Can you work these out from the model? Positions are in its coordinate system, mm. A direction names the side the tool comes from. Round coordinates to 2 decimals unless told otherwise and drop trailing zeros. Order: outer loops, then holes, each group sorted by start corner. A loop starts at its lowest first (then second) coordinate and runs counter-clockwise, first axis right, second up. Notation, with made-up numbers: (-4.75, -30) -> (2.25, -30) arc R14 ccw to (2.25, -10) -> close; hole circle Ø10 at (35.25, -13). An arc over 180 degrees is marked (long way). Use a Markdown table: item, result. Add a question column.
Q1. We'd pull the mould along X, two halves only. Please class faces 3 (the face through (0, -10, 2)), 4 (the face through (-42.15, 11.99, 2.41)), 5 (the face through (4, 15, 2)): +X half, -X half, draft (parallel to the pull), parting line (faces both ways), or undercut.
Q2. For faces 1 (the face through (45, 0, 2)), 2 (the face through (-19.25, 0, 2)), which set-ups out of +Z, -Z, +X, -X, +Y, -Y let a thin tool reach every point of the face, with its end or its side?
Q3. If we section it at B-B on z = 1.5: Give the number of separate pieces and of enclosed holes in the cut face, plus the area to 3 significant figures.
Q4. I need wall thicknesses on line 1 along Y through (x, z) = (37.5, 1.5); line 2 along Y through (x, z) = (24.56, 3.4); line 3 along X through (y, z) = (9.5, 3.2). Which ranges of each line are inside material? Lowest first, please. Write a range as [from, to].
Q5. If we section it at A-A on x = 16: List the corners of the cut face in (y, z) for me, plus the area to 3 significant figures.
```python
from build123d import *

# Parameters (mm, degrees)
ESQUISSE1_W             = 90
ESQUISSE1_H             = 30
BOSS_EXTRU_1_DEPTH      = 4.7625
CONG_1_R                = 10
ESQUISSE2_R             = 6.35
ENL_V_MAT_EXTRU_1_DEPTH = 6
ENL_V_MAT_EXTRU_2_REACH = 49.673
ESQUISSE3_W             = 40
ESQUISSE3_H             = 20
CONG_2_R                = 1.27
ENL_V_MAT_EXTRU_3_REACH = 49.673
ESQUISSE4_R             = 1.09
ENL_V_MAT_EXTRU_4_REACH = 49.673
ESQUISSE6_R             = 1.5


with BuildPart() as part:
    # Esquisse1 → Boss.-Extru.1 (new body)
    with BuildSketch(Plane.XY):
        Rectangle(ESQUISSE1_W, ESQUISSE1_H)
    extrude(amount=BOSS_EXTRU_1_DEPTH)

    # Congé1
    cong_1_edges = [part.edges().sort_by_distance(p)[0] for p in [
        (-45, -15, 2.38125),
        (-45, 15, 2.38125),
    ]]
    fillet(cong_1_edges, radius=CONG_1_R)

    # Esquisse2 → Enlèv. mat.-Extru.1 (cut)
    with BuildSketch(Plane.XY.offset(4.7625)):
        with Locations((-35, 0)):
            Circle(ESQUISSE2_R)
    extrude(amount=-ENL_V_MAT_EXTRU_1_DEPTH, mode=Mode.SUBTRACT)

    # Esquisse3 → Enlèv. mat.-Extru.2 (cut, up to next)
    with BuildSketch(Plane.XY.offset(4.7625), mode=Mode.PRIVATE) as enl_v_mat_extru_2_sk1:
        with Locations((0.75, 0)):
            Rectangle(ESQUISSE3_W, ESQUISSE3_H)
    enl_v_mat_extru_2_tool1 = extrude(enl_v_mat_extru_2_sk1.sketch, amount=-ENL_V_MAT_EXTRU_2_REACH, mode=Mode.PRIVATE) & part.part
    add(enl_v_mat_extru_2_tool1.solids().sort_by_distance((0.75, 0, 4.7625))[0], mode=Mode.SUBTRACT)

    # Congé2
    cong_2_edges = [part.edges().sort_by_distance(p)[0] for p in [
        (-19.25, -10, 2.38125),
        (-19.25, 10, 2.38125),
        (20.75, 10, 2.38125),
        (20.75, -10, 2.38125),
    ]]
    fillet(cong_2_edges, radius=CONG_2_R)

    # Esquisse4 → Enlèv. mat.-Extru.3 (cut, up to next)
    with BuildSketch(Plane.XY.offset(4.7625), mode=Mode.PRIVATE) as enl_v_mat_extru_3_sk1:
        with Locations((-23.06, 5.19)):
            Circle(ESQUISSE4_R)
    enl_v_mat_extru_3_tool1 = extrude(enl_v_mat_extru_3_sk1.sketch, amount=-ENL_V_MAT_EXTRU_3_REACH, mode=Mode.PRIVATE) & part.part
    # Esquisse4 → Enlèv. mat.-Extru.3 (cut, up to next)
    with BuildSketch(Plane.XY.offset(4.7625), mode=Mode.PRIVATE) as enl_v_mat_extru_3_sk2:
        with Locations((-23.06, -5.19)):
            Circle(ESQUISSE4_R)
    enl_v_mat_extru_3_tool2 = extrude(enl_v_mat_extru_3_sk2.sketch, amount=-ENL_V_MAT_EXTRU_3_REACH, mode=Mode.PRIVATE) & part.part
    # Esquisse4 → Enlèv. mat.-Extru.3 (cut, up to next)
    with BuildSketch(Plane.XY.offset(4.7625), mode=Mode.PRIVATE) as enl_v_mat_extru_3_sk3:
        with Locations((24.56, -5.19)):
            Circle(ESQUISSE4_R)
    enl_v_mat_extru_3_tool3 = extrude(enl_v_mat_extru_3_sk3.sketch, amount=-ENL_V_MAT_EXTRU_3_REACH, mode=Mode.PRIVATE) & part.part
    # Esquisse4 → Enlèv. mat.-Extru.3 (cut, up to next)
    with BuildSketch(Plane.XY.offset(4.7625), mode=Mode.PRIVATE) as enl_v_mat_extru_3_sk4:
        with Locations((24.56, 5.19)):
            Circle(ESQUISSE4_R)
    enl_v_mat_extru_3_tool4 = extrude(enl_v_mat_extru_3_sk4.sketch, amount=-ENL_V_MAT_EXTRU_3_REACH, mode=Mode.PRIVATE) & part.part
    add(enl_v_mat_extru_3_tool1.solids().sort_by_distance((-23.06, 5.19, 4.7625))[0], mode=Mode.SUBTRACT)
    add(enl_v_mat_extru_3_tool2.solids().sort_by_distance((-23.06, -5.19, 4.7625))[0], mode=Mode.SUBTRACT)
    add(enl_v_mat_extru_3_tool3.solids().sort_by_distance((24.56, -5.19, 4.7625))[0], mode=Mode.SUBTRACT)
    add(enl_v_mat_extru_3_tool4.solids().sort_by_distance((24.56, 5.19, 4.7625))[0], mode=Mode.SUBTRACT)

    # Esquisse6 → Enlèv. mat.-Extru.4 (cut, up to next)
    with BuildSketch(Plane.XY.offset(4.7625), mode=Mode.PRIVATE) as enl_v_mat_extru_4_sk1:
        with Locations((37.5, 10)):
            Circle(ESQUISSE6_R)
    enl_v_mat_extru_4_tool1 = extrude(enl_v_mat_extru_4_sk1.sketch, amount=-ENL_V_MAT_EXTRU_4_REACH, mode=Mode.PRIVATE) & part.part
    # Esquisse6 → Enlèv. mat.-Extru.4 (cut, up to next)
    with BuildSketch(Plane.XY.offset(4.7625), mode=Mode.PRIVATE) as enl_v_mat_extru_4_sk2:
        with Locations((37.5, -10)):
            Circle(ESQUISSE6_R)
    enl_v_mat_extru_4_tool2 = extrude(enl_v_mat_extru_4_sk2.sketch, amount=-ENL_V_MAT_EXTRU_4_REACH, mode=Mode.PRIVATE) & part.part
    add(enl_v_mat_extru_4_tool1.solids().sort_by_distance((37.5, 10, 4.7625))[0], mode=Mode.SUBTRACT)
    add(enl_v_mat_extru_4_tool2.solids().sort_by_distance((37.5, -10, 4.7625))[0], mode=Mode.SUBTRACT)


solid = part.part
```
Answer below:
| question | item | result |
|---|---|---|
| 1 | face 3 | undercut |
| 1 | face 4 | -X half |
| 1 | face 5 | draft |
| 2 | face 1 | +Z, -Z, +X, +Y, -Y |
| 2 | face 2 | +Z, -Z |
| 3 | separate pieces | 1 |
| 3 | enclosed holes | 8 |
| 3 | area | 1,700 mm² |
| 4 | line 1 | [-15, -11.5], [-8.5, 8.5], [11.5, 15] |
| 4 | line 2 | [-15, -6.28], [-4.1, 4.1], [6.28, 15] |
| 4 | line 3 | [-43.93, -18.99], [20.49, 36.09], [38.91, 45] |
| 5 | outline | (-15, 0) -> (-10, 0) -> (-10, 4.76) -> (-15, 4.76) -> close; (10, 0) -> (15, 0) -> (15, 4.76) -> (10, 4.76) -> close |
| 5 | area | 47.6 mm² |
